Input: part model. Units: mm. Frame: model coordinates. A direction names the side the tool comes from. Round coordinates to 2 decimals unless told otherwise and drop trailing zeros. Loops run counter-clockwise (first coordinate to the right, second up) from the corner with the lowest first, then second, coordinate; pieces in that order, holes last.
1) Draft query along Y for faces 4 (the face through (-6.095, -22.92, 0.789)), 5 (the face through (-6.695, -18.793, 0.789)), 6 (the face through (8, 23, 0)). Return one class per face: pulls with the +Y half, pulls with the -Y half, needs draft (parallel to the pull), parting line crosses it, or undercut.
2) Section D-D, the plane x = 0. Return loops of the section in (y, z).
3) Section C-C, the plane x = -17. Return loops of the section in (y, z).
4) Access query for faces 1 (the face through (6.095, -22.92, 0.789)), 2 (the face through (8, 23, 1.6)), 3 (the face through (10.43, -19.93, 0.79)). Directions: +Z, -Z, +X, -X, +Y, -Y. A direction counts if a zero-diameter tool reaches every point of the face in a straight line with its end or side. Return the directions, or none.
5) Ray query, line 1 along Y through (x, z) = (-8.5, 1.4); line 2 along Y through (x, z) = (9, 0.95); line 3 along X through (y, z) = (-21, 1.5). Return the intervals inside material, ascending.
6) Section B-B, the plane z = 1.15. Return loops of the section in (x, y).
7) Section A-A, the plane y = -16.5. Return loops of the section in (x, z), and give its area (3 significant figures).
Autodesk Inventor part; units mm, degrees
ref_plane "WorkPlane1" through (0, 0, 0) normal (0, 0, 1) x (1, 0, 0)
ref_plane "Work Plane2" through (0, 0, -1.6) normal (0, 0, 1) x (1, 0, 0)
ref_plane "WorkPlane2" through (0, 0, 1) normal (0, 0, 1) x (1, 0, 0)
ref_plane "WorkPlane1" through (0, 0, 0) normal (0, 0, 1) x (1, 0, 0)
ref_plane "Work Plane2" through (0, 0, -1.6) normal (0, 0, 1) x (1, 0, 0)
ref_plane "WorkPlane2" through (0, 0, 1) normal (0, 0, 1) x (1, 0, 0)
sketch "Sketch1" plane through (0, 0, 0) normal (0, 0, 1) x (1, 0, 0)
  point P0 (0, 0)
sketch "Sketch2" plane through (0, 0, 0) normal (0, 0, 1) x (1, 0, 0)
  line L0 (6.5, -24.5254) -> (5.6777, -21.2687)
  arc A0 (9.3003, -18.9899) -> (5.6777, -21.2687) centre (7.8592, -20.7178) ccw
  line L1 (9.3003, -18.9899) -> (11.5824, -20.8932)
  arc A1 (11.5824, -20.8932) -> (-11.5824, -20.8932) centre (0, 0) ccw
  line L2 (-9.3003, -18.9899) -> (-11.5824, -20.8932)
  arc A2 (-5.6777, -21.2687) -> (-9.3003, -18.9899) centre (-7.8592, -20.7178) ccw
  line L3 (-6.5, -24.5254) -> (-5.6777, -21.2687)
  arc A3 (6.5, -24.5254) -> (-6.5, -24.5254) centre (0, 1.2167) ccw
  line L4 (0, 1.2167) -> (-6.5, -24.5254) construction
  line L5 (0, 1.2167) -> (6.5, -24.5254) construction
  dimension "d2" = 26.55
  dimension "d4" = 0
  dimension "d6" = 23.8889
  dimension "d8" = 1.2167
  dimension "d10" = 6.5
  dimension "d12" = 6.5
  dimension "d14" = 2.25
  dimension "d16" = 2.25
  dimension "d18" = 23.3
  dimension "d20" = 23.3
  dimension "d22" = 36
  dimension "d24" = 36
extrude "Extrusion1" add sketch "Sketch2" along normal blind 1.6
sketch "Sketch3" plane through (0, 0, 1.6) normal (0, 0, 1) x (1, 0, 0)
  arc A0 (-5.6777, -21.2687) -> (-9.3003, -18.9899) centre (-7.8592, -20.7178) ccw
hole "Hole1" at (-7.8592, -20.7178, 1.6) direction (0, 0, -1) diameter 2.5 end through all
sketch "Sketch4" plane through (0, 0, 1.6) normal (0, 0, 1) x (1, 0, 0)
  arc A0 (9.3003, -18.9899) -> (5.6777, -21.2687) centre (7.8592, -20.7178) ccw
hole "Hole2" at (7.8592, -20.7178, 1.6) direction (0, 0, -1) diameter 2.5 end through all
equation "\"d29\" = Diam5"
equation "\"d36\" = Diam5"
equation "\"d2\" = 0.5 * Diam2"
equation "\"d6\" = 0.5 * msp_dd1"
equation "\"d8\" = -0.5 * msp_dd1 + 0.5 * Diam2 - 0.222222 * ParA"
equation "\"d10\" = 2.6 * Diam5"
equation "\"d12\" = 2.6 * Diam5"
equation "\"d14\" = 0.9 * Diam5"
equation "\"d16\" = 0.9 * Diam5"
equation "\"d18\" = 1.3 * Diam5 + 0.5 * Diam2 - ParA"
equation "\"d20\" = 1.3 * Diam5 + 0.5 * Diam2 - ParA"
equation "\"d25\" = ParS"
equation "\"Diam5\" = 2.5"
equation "\"ParA\" = 6.5"
equation "\"ParS\" = 1.6"
equation "\"Diam2\" = 53.1"
equation "\"msp_dd1\" = -b + Diam2 - 0.111111 * ParA"
equation "\"msp_pom\" = 0.5 * Diam2 - b"
equation "\"TEMPLATE\" = 1.2345"
properties part number "ANSI B 27.7M - 3BMI-50" material "Steel, Mild"
Final values:
1. face 4: pulls with the -Y half
1. face 5: undercut
1. face 6: needs draft
2. outline: (23.89, 0) - (27.77, 0) - (27.77, 1.6) - (23.89, 1.6) - close
3. outline: (-19.18, 0) - (-16.78, 0) - (-16.78, 1.6) - (-19.18, 1.6) - close; (16.78, 0) - (21.61, 0) - (21.61, 1.6) - (16.78, 1.6) - close
4. face 1: +Z, -Z, -Y
4. face 2: +Z, +X, -X, +Y, -Y
4. face 3: +Z, -Z
5. line 1: y = -23.94 to -21.79, -19.64 to -18.56, 22.33 to 26.37
5. line 2: y = -23.76 to -21.23, -20.21 to -18.78, 22.13 to 26.19
5. line 3: x = -14.54 to -9.08, -6.64 to -5.63, 5.63 to 6.64, 9.08 to 14.54
6. outline: (-11.58, -20.89) arc R23.89 cw (long way) to (11.58, -20.89) - (9.3, -18.99) arc R2.25 ccw to (5.68, -21.27) - (6.5, -24.53) arc R26.55 ccw (long way) to (-6.5, -24.53) - (-5.68, -21.27) arc R2.25 ccw to (-9.3, -18.99) - close; hole circle Ø2.5 at (-7.86, -20.72); hole circle Ø2.5 at (7.86, -20.72)
7. outline: (-19.77, 0) - (-17.28, 0) - (-17.28, 1.6) - (-19.77, 1.6) - close; (17.28, 0) - (19.77, 0) - (19.77, 1.6) - (17.28, 1.6) - close
7. area: 8.00 mm2
